```python
from build123d import *

# Parameters (mm, degrees)
SKETCH1_R           = 3
BOSS_EXTRUDE1_DEPTH = 21.8
CUT_EXTRUDE2_START  = -12
CUT_EXTRUDE2_DEPTH  = 12
FILLET1_R           = 0.5


with BuildPart() as part:
    # Sketch1 → Boss-Extrude1 (new body)
    with BuildSketch(Plane(origin=(0, 0, 0), x_dir=(0, 0, -1), z_dir=(1, 0, 0))):
        Circle(SKETCH1_R)
    extrude(amount=BOSS_EXTRUDE1_DEPTH)

    # Sketch2 → Cut-Extrude2 (cut)
    with BuildSketch(Plane(origin=(21.8, 0, 0), x_dir=(0, 0, -1), z_dir=(1, 0, 0)).offset(CUT_EXTRUDE2_START)):
        with BuildLine():
            Line((0, -2.5), (-1.658312395, -2.5))
            ThreePointArc((-1.658312395, -2.5), (0, -3), (1.658312395, -2.5))
            Line((1.658312395, -2.5), (0, -2.5))
        make_face()
    extrude(amount=CUT_EXTRUDE2_DEPTH, mode=Mode.SUBTRACT)

    # Fillet1
    fillet1_edges = [part.edges().sort_by_distance(p)[0] for p in [
        (21.8, 2.643382037, 1.418637165),
        (21.8, -2.5, 0),
    ]]
    fillet(fillet1_edges, radius=FILLET1_R - 0.0001)  # a hair under: the kernel refuses the full size


solid = part.part
```
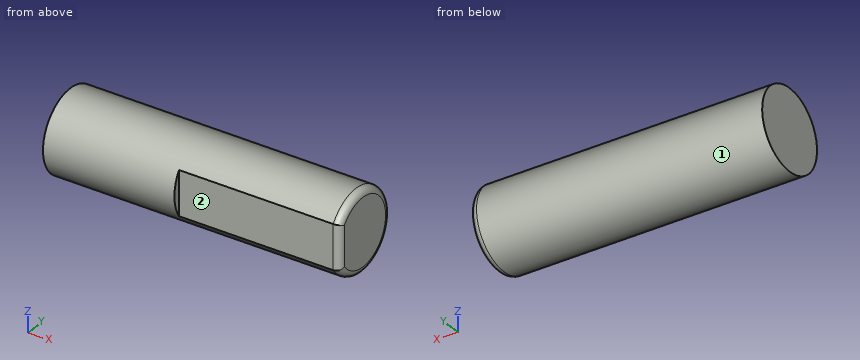
Geometry: final body of the model. Coordinates: model frame, mm. Face numbers are marked on the shaded views. A direction names the side the tool comes from. Coordinates: 2 decimals unless noted, no trailing zeros. Order: outer loops, then holes, each group sorted by start corner. A loop starts at its lowest first (then second) coordinate and runs counter-clockwise, first axis right, second up. Notation, with made-up numbers: (32, 61.5) -> (82, 61.5) arc R28 cw to (82, 96.5) -> close; hole circle Ø6 at (-8, -18). An arc over 180 degrees is marked (long way). Use CSV: the item, a comma, the result in double quotes.
1) Section C-C on x = 15.25. Output: boundary loops of the cut face in (y, z).
Findings:
outline,"(-2.5, -1.66) arc R3 ccw (long way) to (-2.5, 1.66) -> close"
2) Access query for the marked faces 1 and 2. Directions: +Z, -Z, +X, -X, +Y, -Y. A direction counts if a zero-diameter tool reaches every point of the face in a straight line with its end or side. Return the directions, or none.
Findings:
face 1,"+X, -X"
face 2,"+Z, -Z, +X, -Y"
3) Section B-B on x = 8.75. Output: boundary loops of the cut face in (y, z).
Findings:
outline,"circle Ø6 at (0, 0)"
4) Section A-A on z = 0. Output: boundary loops of the cut face in (x, y).
Findings:
outline,"(0, -3) -> (9.8, -3) -> (9.8, -2.5) -> (21.3, -2.5) arc R0.5 ccw to (21.8, -2) -> (21.8, 2.5) arc R0.5 ccw to (21.3, 3) -> (0, 3) -> close"
5) Pin query (flat end, axial travel): pin 1 Ø0.6 at (y, z) = (-2.5, 0.5) entering from +X; pin 2 Ø3 at (x, y) = (19, -2.5) entering from +Z; pin 3 Ø1 at (x, y) = (8, 2) entering from +Z. Return the tip coordinate at first contact, or that it passes through.
Findings:
pin 1,"stops at x = 21.76"
pin 2,"stops at z = 2.83"
pin 3,"stops at z = 2.6"
6) Line query: line 1 (Y direction, x = 11.5, z = -2.5); line 2 (Y direction, x = 13.25, z = -1.5); line 3 (X direction, y = 2.5, z = 0.5). Output: solid intervals per line, ascending.
Findings:
line 1,"y = -1.66 to 1.66"
line 2,"y = -2.5 to 2.6"
line 3,"x = 0 to 21.8"
